from build123d import *

# Parameters (mm, degrees)
F1_DEPTH      = 35
F3_DEPTH      = 4.001
F5_DEPTH      = 2.3104010768
F5_DEPTH_BACK = 2.3104010768


with BuildPart() as f1:
    # F0 (on Front) → F1 (new body)
    with BuildSketch(Plane.XZ):
        Polygon((-6.6223553988, -1.1547005384), (-6.6223553988, 1.1547005384), (-8.6223553988, 2.3094010768), (-10.6223553988, 1.1547005384), (-10.6223553988, -1.1547005384), (-8.6223553988, -2.3094010768), align=None)
    extrude(amount=F1_DEPTH)

    # F2 (on face) → F3 (cut, through all)
    with BuildSketch(Plane.YZ.offset(-6.6223553988)):
        Polygon((-35, 2.5), (-35, 0), (-25, 2.5), align=None)
        Polygon((-25, -2.5), (-35, 0), (-35, -2.5), align=None)
    extrude(amount=-F3_DEPTH, mode=Mode.SUBTRACT)

    # F4 (on Top) → F5 (cut, two sides)
    with BuildSketch(Plane.XY) as f5_sk:
        Polygon((-6.6223553988, -35), (-6.6223553988, -30.3811978465), (-7.6223553988, -35), align=None)
        Polygon((-10.6223553988, -35), (-9.6223553988, -35), (-10.6223553988, -30.3811978465), align=None)
    extrude(amount=-F5_DEPTH, mode=Mode.SUBTRACT)
    extrude(f5_sk.sketch, amount=F5_DEPTH_BACK, mode=Mode.SUBTRACT)


solid = f1.part
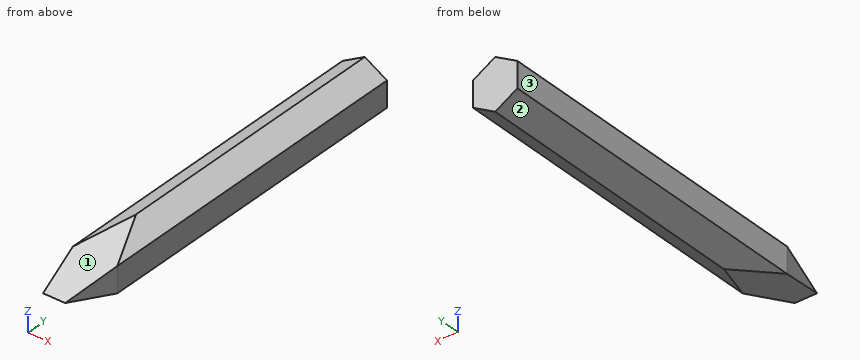
The model under review builds one solid part; all positions refer to its coordinate system, in mm. Face numbers are marked on the shaded views. Round coordinates to 2 decimals unless told otherwise and drop trailing zeros. Write each loop counter-clockwise with the first axis right and the second up, starting at its lowest first coordinate (ties: lowest second). Pieces come first, ordered by that corner, then holes. Notation, with made-up numbers: (-26, 39) - (32, 39) arc R22 ccw to (32, 56) - close; hole circle Ø4 at (5, -33). An arc over 180 degrees is marked (long way). One line per item, written item: value. Start each with the question number.
1. Consider section B-B on x = -9.25. Write out the cut boundary in (y, z), and give its area (3 significant figures).
2. The part is to be moulded in two halves that separate along Z. For the marked faces 1, 2 and 3, say which applies: released by +Z, released by -Z, zero draft, split by the parting line, or undercut.
3. Consider section C-C on z = -0.5. Write out the cut boundary in (x, y).
4. To check wall thickness, follow L1, parallel to X at y = -23.5, z = -1.7; L2, parallel to Z at x = -7.1, y = -21; L3, parallel to Z at x = -10.3, y = -25. State the ranges of each line that lie inside material, in increasing order. Write a range as from..to.
5. Consider section D-D on y = -4. Write out the cut boundary in (x, z), and give its area (3 significant figures).
6. Consider section A-A on y = -28.5. Write out the cut boundary in (x, z) (3 decimals), and give its area (3 significant figures).
Checks:
1. outline: (-35, 0) - (-27.21, -1.95) - (0, -1.95) - (0, 1.95) - (-27.21, 1.95) - close
1. area: 121 mm^2
2. face 1: released by +Z
2. face 2: released by -Z
2. face 3: zero draft
3. outline: (-10.62, -30.38) - (-10.06, -33) - (-7.19, -33) - (-6.62, -30.38) - (-6.62, 0) - (-10.62, 0) - close
4. L1: x = -9.68..-7.57
4. L2: z = -1.43..1.43
4. L3: z = -1.34..1.34
5. outline: (-10.62, -1.15) - (-8.62, -2.31) - (-6.62, -1.15) - (-6.62, 1.15) - (-8.62, 2.31) - (-10.62, 1.15) - close
5. area: 13.9 mm^2
6. outline: (-10.622, -1.155) - (-9.808, -1.625) - (-7.437, -1.625) - (-6.622, -1.155) - (-6.622, 1.155) - (-7.437, 1.625) - (-9.808, 1.625) - (-10.622, 1.155) - close
6. area: 12.2 mm^2
